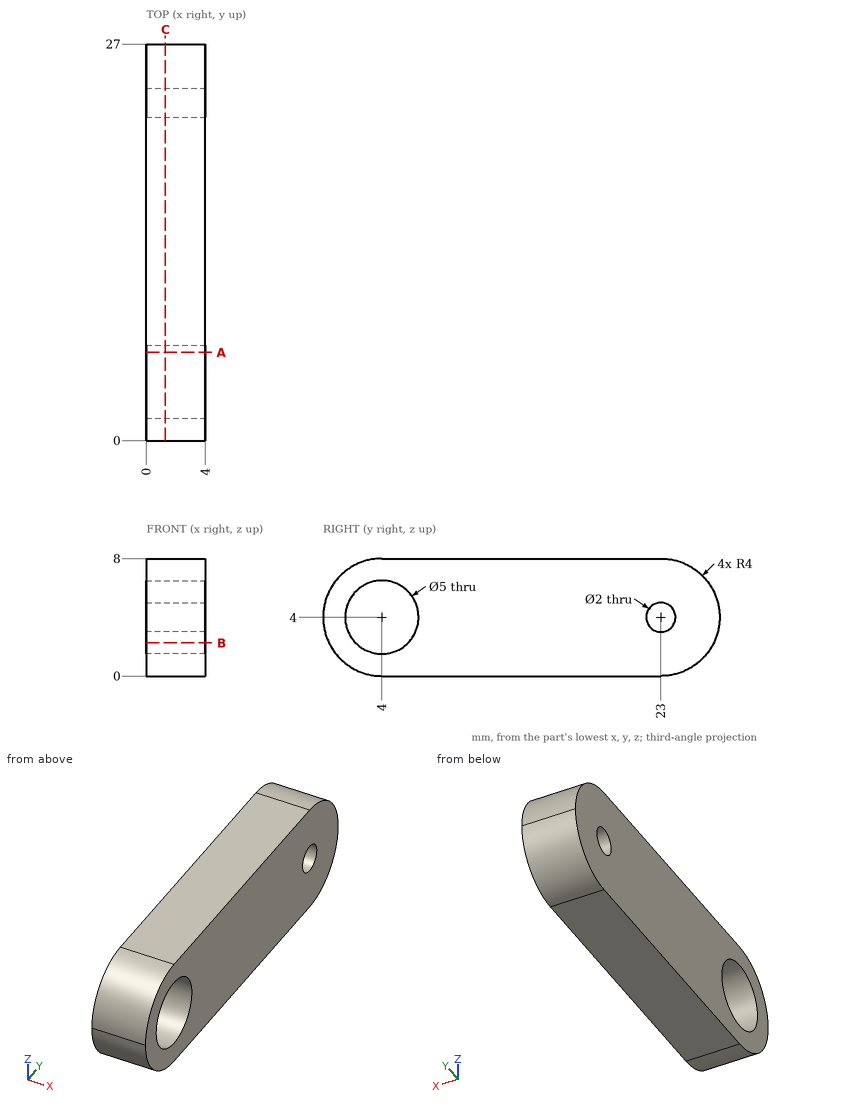
Job drawing, mm, ordinate dimensions from the low corner. One solid piece. Give positions to 0.01 mm unless a question says otherwise; leave off trailing zeros. Order: outer loops, then holes, each group sorted by start corner. A loop starts at its lowest first (then second) coordinate and runs counter-clockwise, first axis right, second up. Notation, with made-up numbers: M -34.75,50.5 L -22.75,50.5 A22 ccw -22.75,67.5 Z; hole C 30.25,63 d11. An arc over 180 degrees is marked long. Return JSON: item names as keys, results as strings.
Q1. Flat gauge pins, fed straight in: pin 1 (2 mm diameter, centred on x = 2.5, y = 13.5, fed in from -Z); pin 2 (1.8 mm diameter, centred on y = 23, z = 4, fed in from -X); pin 3 (1 mm diameter, centred on x = 0.5, z = 2, fed in from +Y); pin 4 (2 mm diameter, centred on x = 1, z = 6, fed in from +Y). Where does each tip first touch, or does it go through?
Answer list:
{"pin 1": "stops at z = 0", "pin 2": "passes through", "pin 3": "stops at y = 26.71", "pin 4": "stops at y = 26.87"}
Q2. Band-saw the part on B-B (z = 2.25). Give the cut face in (x, y), then the cut area to 3 significant figures.
Answer list:
{"outline": "M 0,0.4 L 4,0.4 L 4,2.21 L 0,2.21 Z; M 0,5.79 L 4,5.79 L 4,26.6 L 0,26.6 Z", "area": "90.5 mm^2"}
Q3. Wall check: probe 1 along Y at (x, z) = (2.75, 4); probe 2 along Z at (x, y) = (3.7, 3.75); probe 3 along Z at (x, y) = (0.55, 5). Give the ranges that are in metal, low to high. Write a range as from..to.
Answer list:
{"probe 1": "y = 0..1.5, 6.5..22, 24..27", "probe 2": "z = 0.01..1.51, 6.49..7.99", "probe 3": "z = 0..1.71, 6.29..8"}
Q4. Band-saw the part on C-C (x = 1.3). Count the separate pieces of the cut face and the enclosed holes in it, then the cut area to 4 significant figures.
Answer list:
{"separate pieces": "1", "enclosed holes": "2", "area": "179.5 mm^2"}
Q5. Band-saw the part on A-A (y = 6). Give the cut face in (x, z), then the cut area to 3 significant figures.
Answer list:
{"outline": "M 0,0 L 4,0 L 4,2.5 L 0,2.5 Z; M 0,5.5 L 4,5.5 L 4,8 L 0,8 Z", "area": "20.0 mm^2"}
